Verification items for the finished model (mm, model axes). A direction names the side the tool comes from. Coordinates: 2 decimals unless noted, no trailing zeros. Write each loop counter-clockwise with the first axis right and the second up, starting at its lowest first coordinate (ties: lowest second). Pieces come first, ordered by that corner, then holes. Notation, with made-up numbers: (7.25, -18.75) -> (12.25, -18.75) arc R9 cw to (12.25, -6.75) -> close; hole circle Ø5 at (4, -23.75). An arc over 180 degrees is marked (long way). Write item = value, one per line. Start each with the question number.
(1) Section check A-A (z = 4.25). State how many separate pieces and enclosed holes the cut face has, plus the area to 3 significant figures.
(2) Section check C-C (y = -21). Record the cut outline in (x, z), plus the area to 3 significant figures.
(3) Gauge pin test, flat ends, axial feed: pin 1 Ø1.5 at (y, z) = (-91, 5.5) entering from -X; pin 2 Ø6.5 at (x, y) = (-105.15, -59.25) entering from -Z; pin 3 Ø2 at (x, z) = (-8.5, 5.5) entering from +Y; pin 4 Ø3 at (y, z) = (-80, 5) entering from +X. Record the tip position at first contact, or that the pin passes through.
(4) Section check B-B (x = 103.5). Record the cut outline in (y, z), plus the area to 3 significant figures.
(5) Material ranges on probe 1 along Y at (x, z) = (0.5, 3.75); probe 2 along X at (y, z) = (71, 4); probe 3 along X at (y, z) = (2, 3), recorded low to high. Write a range as [from, to].
(6) Mould release check, pull along Y, two halves, no side actions. Record for faces 3 (the face through (39.956, -35.634, 3.219)), 4 (the face through (21, -19, 0)), 5 (the face through (-103.316, -62.771, 3.219)), 6 (the face through (-94.226, -78.119, 3.131)): released by +Y, released by -Y, zero draft, split by the parting line, or undercut.
(7) Set-up check for faces 1 (the face through (-0.59, 4.46, 3.22)), 2 (the face through (-48.17, -93.9, 3.22)): record each of +Z, -Z, +X, -X, +Y, -Y from which the full face is reachable in a straight line by a thin tool's end or side.
```python
from build123d import *

# Parameters (mm, degrees)
BOSS_EXTRUDE2_DEPTH = 6.35
CUT_EXTRUDE1_DEPTH  = 7.3500001
BOSS_EXTRUDE3_DEPTH = 6.35
SKETCH10_R          = 3.96875
CUT_EXTRUDE2_DEPTH  = 7.35
SKETCH11_R          = 4.5
CUT_EXTRUDE4_DEPTH  = 7.35
BOSS_EXTRUDE4_DEPTH = 6.35
SKETCH13_R          = 1.75
CUT_EXTRUDE5_DEPTH  = 7.35
LPATTERN1_COUNT     = 2
LPATTERN1_PITCH     = 64
SKETCH14_R          = 2.54
CUT_EXTRUDE6_DEPTH  = 7.35
SKETCH15_R          = 1.75
CUT_EXTRUDE7_DEPTH  = 7.35
SKETCH16_R          = 1.75
CUT_EXTRUDE8_DEPTH  = 7.35
SKETCH17_R          = 1.75
CUT_EXTRUDE9_DEPTH  = 7.35
SKETCH19_R          = 3.96875
CUT_EXTRUDE11_DEPTH = 7.35
SKETCH21_R          = 2.54
CUT_EXTRUDE12_DEPTH = 7.35
SKETCH22_R          = 3.96875
CUT_EXTRUDE13_DEPTH = 7.35
SKETCH23_R          = 4.885116726
SKETCH23_R_2        = 5.670398183
BOSS_EXTRUDE5_DEPTH = 6.35
CUT_EXTRUDE14_DEPTH = 7.35
FILLET1_R           = 3.175


with BuildPart() as part:
    # Sketch6 → Boss-Extrude2 (new body)
    with BuildSketch(Plane.XY):
        with BuildLine():
            Line((-68.006850091, -76.67090114), (-109.486767671, -48.656527855))
            Line((-109.486767671, -48.656527855), (-118.371760678, -61.812230963))
            Line((-118.371760678, -61.812230963), (18.447551645, -154.216158235))
            Line((18.447551645, -154.216158235), (135.729459338, 19.43912279))
            Line((135.729459338, 19.43912279), (-1.089852986, 111.843050063))
            Line((-1.089852986, 111.843050063), (-73.946795643, 3.966284577))
            Line((-73.946795643, 3.966284577), (-56.624438948, -7.732749433))
            ThreePointArc((-56.624438948, -7.732749433), (-43.058385537, 37.577891571), (0, 57.15))
            ThreePointArc((0, 57.15), (56.404848571, 31.095576642), (70.829334649, -29.338471048))
            add(Edge.make_bspline(
                [(70.829334649, -29.338471048), (70.811686062, -29.418295928), (70.776015112, -29.578104383), (70.713320217, -29.85478305), (70.619021771, -30.262929245), (70.501052001, -30.762086912), (70.364034474, -31.322191481), (70.199318515, -31.970958926), (70.000453855, -32.723919765), (69.795103485, -33.469783355), (69.582015398, -34.214296028), (69.361377803, -34.956693289), (69.133257682, -35.696762218), (68.838782679, -36.61892651), (68.470566207, -37.720710028), (68.019498024, -38.998776477), (67.474836154, -40.448808619), (66.901337925, -41.887676852), (66.299328392, -43.31485223), (65.669141732, -44.729810424), (65.011119088, -46.132040323), (64.325609411, -47.52103904), (63.612968547, -48.896314904), (62.87355937, -50.257385735), (62.107751613, -51.603779381), (61.315921169, -52.935034173), (60.49845004, -54.250698756), (59.655726138, -55.550331897), (58.571247582, -57.154294757), (57.220953058, -59.045283389), (55.576035723, -61.200397094), (53.604026134, -63.590264702), (51.54329346, -65.904053004), (49.39728314, -68.138962994), (47.169496434, -70.29235602), (44.863486103, -72.361752995), (42.482847363, -74.344831806), (40.031215607, -76.239428526), (36.882516177, -78.494556171), (32.976808929, -81.016011003), (28.250788286, -83.68089187), (21.41551215, -86.919136497), (14.30829026, -89.526654921), (6.996956895, -91.488176442), (-0.451922312, -92.797413176), (-6.61686174, -93.456358442), (-12.81195397, -93.702029749), (-19.009644204, -93.537285056), (-25.183124422, -92.966685286), (-31.306438312, -91.996382122), (-36.598524037, -90.804323442), (-41.072542301, -89.543185606), (-44.752319298, -88.33589156), (-47.664184976, -87.27761875), (-50.541347258, -86.128353728), (-53.381128552, -84.889612663), (-56.180924218, -83.562977818), (-58.593536599, -82.326710176), (-60.633378351, -81.214215821), (-62.313751085, -80.252471782), (-63.646071553, -79.462491566), (-64.966093336, -78.652178853), (-66.222359154, -77.854259082), (-67.143044791, -77.250601571), (-67.736251212, -76.85365602), (-68.006850091, -76.67090114)],
                knots=[0.071020771, 0.071020771, 0.071020771, 0.071020771, 0.071020771, 0.072848477, 0.074676184, 0.07650389, 0.078331597, 0.08198701, 0.085642423, 0.089297836, 0.092953249, 0.096608662, 0.100264075, 0.103919488, 0.107574901, 0.114885727, 0.122196554, 0.12950738, 0.136818214, 0.144129048, 0.151439882, 0.158750716, 0.166061558, 0.173372401, 0.180683243, 0.187994085, 0.195304924, 0.202615763, 0.209926602, 0.217237441, 0.231859103, 0.246480766, 0.261102426, 0.275724085, 0.290345754, 0.304967424, 0.319589099, 0.334210774, 0.348832457, 0.36345414, 0.392697464, 0.421940789, 0.451184112, 0.506140643, 0.535383973, 0.564627303, 0.593870641, 0.623113979, 0.652357319, 0.68160066, 0.710843985, 0.740087309, 0.754708984, 0.769330659, 0.783952333, 0.798574008, 0.813195669, 0.82781733, 0.842438991, 0.849749821, 0.857060652, 0.86437149, 0.871682327, 0.878993165, 0.885158103, 0.885158103, 0.885158103, 0.885158103, 0.885158103], degree=4))
        make_face()
    extrude(amount=BOSS_EXTRUDE2_DEPTH)

    # Sketch8 → Cut-Extrude1 (cut, through all)
    with BuildSketch(Plane.XY.offset(6.35)):
        Polygon((-71.011229489, -93.798205788), (-53.378672597, -90.381637707), (-42.854110111, -97.489632113), (-39.43754203, -115.122189004), align=None)
    extrude(amount=-CUT_EXTRUDE1_DEPTH, mode=Mode.SUBTRACT)

    # Sketch9 → Boss-Extrude3 (add, through all)
    with BuildSketch(Plane.XY.offset(6.35)):
        Polygon((-1.089852986, 111.843050063), (-109.486767671, -48.656527855), (27.332544652, -141.060455127), (135.729459338, 19.43912279), align=None)
    extrude(amount=-BOSS_EXTRUDE3_DEPTH)

    # Sketch10 → Cut-Extrude2 (cut, through all)
    with BuildSketch(Plane.XY.offset(6.35)):
        with Locations((4.996496209, -84.796642912)):
            Circle(SKETCH10_R)
        with Locations((40.816310536, -31.759477627)):
            Circle(SKETCH10_R)
        with Locations((76.636124864, 21.277687659)):
            Circle(SKETCH10_R)
        with Locations((-45.295165913, -45.214466102)):
            Circle(SKETCH10_R)
    extrude(amount=-CUT_EXTRUDE2_DEPTH, mode=Mode.SUBTRACT)

    # Sketch11 → Cut-Extrude4 (cut, through all)
    with BuildSketch(Plane.XY.offset(6.35)):
        Circle(SKETCH11_R)
    extrude(amount=-CUT_EXTRUDE4_DEPTH, mode=Mode.SUBTRACT)

    # Sketch12 → Boss-Extrude4 (add, through all)
    with BuildSketch(Plane.XY.offset(6.35)):
        Polygon((135.729459338, 19.43912279), (67.319803176, 65.641086427), (88.643786393, 97.214773886), (157.053442554, 51.01281025), align=None)
    extrude(amount=-BOSS_EXTRUDE4_DEPTH)

    # Sketch13 → Cut-Extrude5 (cut, through all)
    with BuildSketch(Plane.XY.offset(6.35)):
        with Locations((94.899221836, -29.671127724)):
            Circle(SKETCH13_R)
    cut_extrude5 = extrude(amount=-CUT_EXTRUDE5_DEPTH, mode=Mode.SUBTRACT)

    # LPattern1: Cut-Extrude5 ×2
    with Locations(*[Vector(-0.559684599, -0.828705708, 0) * (i * LPATTERN1_PITCH) for i in range(1, LPATTERN1_COUNT)]):
        add(cut_extrude5, mode=Mode.SUBTRACT)

    # Sketch14 → Cut-Extrude6 (cut, through all)
    with BuildSketch(Plane.XY.offset(6.35)):
        with Locations((71.72703343, -52.635713164)):
            Circle(SKETCH14_R)
        with Locations((35.907219102, -105.67287845)):
            Circle(SKETCH14_R)
        with Locations((115.740620068, 63.589229581)):
            Circle(SKETCH14_R)
    extrude(amount=-CUT_EXTRUDE6_DEPTH, mode=Mode.SUBTRACT)

    # Sketch15 → Cut-Extrude7 (cut, through all)
    with BuildSketch(Plane.XY.offset(6.35)):
        with Locations((-105.147343009, -59.249804902)):
            Circle(SKETCH15_R)
        with Locations((15.885125585, -140.991740566)):
            Circle(SKETCH15_R)
        with Locations((1.472573075, 98.618632394)):
            Circle(SKETCH15_R)
    extrude(amount=-CUT_EXTRUDE7_DEPTH, mode=Mode.SUBTRACT)

    # Sketch16 → Cut-Extrude8 (cut, through all)
    with BuildSketch(Plane.XY.offset(6.35)):
        with Locations((92.060354474, 79.582216994)):
            Circle(SKETCH16_R)
        with Locations((139.420885662, 47.596242169)):
            Circle(SKETCH16_R)
    extrude(amount=-CUT_EXTRUDE8_DEPTH, mode=Mode.SUBTRACT)

    # Sketch17 → Cut-Extrude9 (cut, through all)
    with BuildSketch(Plane.XY.offset(6.35)):
        with Locations((-26.311406216, 17.769986014)):
            Circle(SKETCH17_R)
        with Locations((17.769986014, 26.311406216)):
            Circle(SKETCH17_R)
    extrude(amount=-CUT_EXTRUDE9_DEPTH, mode=Mode.SUBTRACT)

    # Sketch19 → Cut-Extrude11 (cut, through all)
    with BuildSketch(Plane.XY.offset(6.35)):
        with Locations((-65.680233685, -85.904783923)):
            Circle(SKETCH19_R)
    extrude(amount=-CUT_EXTRUDE11_DEPTH, mode=Mode.SUBTRACT)

    # Sketch21 → Cut-Extrude12 (cut, through all)
    with BuildSketch(Plane.XY.offset(6.35)):
        with Locations((-13.666272317, 70.530227577)):
            Circle(SKETCH21_R)
        with Locations((26.00698069, 78.217505758)):
            Circle(SKETCH21_R)
        with Locations((-86.729358658, -71.688795112)):
            Circle(SKETCH21_R)
        with Locations((-8.64928203, -120.590613931)):
            Circle(SKETCH21_R)
    extrude(amount=-CUT_EXTRUDE12_DEPTH, mode=Mode.SUBTRACT)

    # Sketch22 → Cut-Extrude13 (cut, through all)
    with BuildSketch(Plane.XY.offset(6.35)):
        with Locations((-105.147343009, -59.249804902)):
            Circle(SKETCH22_R)
    extrude(amount=-CUT_EXTRUDE13_DEPTH, mode=Mode.SUBTRACT)

    # Sketch23 → Boss-Extrude5 (add, through all)
    with BuildSketch(Plane.XY.offset(6.35)):
        with Locations((-86.729358658, -71.688795112)):
            Circle(SKETCH23_R)
        with Locations((-65.680233685, -85.904783923)):
            Circle(SKETCH23_R_2)
    extrude(amount=-BOSS_EXTRUDE5_DEPTH)

    # Sketch24 → Cut-Extrude14 (cut, through all)
    with BuildSketch(Plane.XY.offset(6.35)):
        Polygon((85.800588631, 93.004948891), (87.167215863, 85.951926135), (71.529628171, 62.797888664), (67.319803176, 65.641086427), align=None)
    extrude(amount=-CUT_EXTRUDE14_DEPTH, mode=Mode.SUBTRACT)

    # Fillet1
    fillet1_edges = [part.edges().sort_by_distance(p)[0] for p in [
        (-1.089852986, 111.843050063, 3.175),
        (18.447551645, -154.216158235, 3.175),
        (-118.371760678, -61.812230963, 3.175),
        (85.800588631, 93.004948891, 3.175),
        (87.167215863, 85.951926135, 3.175),
        (71.529628171, 62.797888664, 3.175),
        (-39.43754203, -115.122189004, 3.175),
        (-71.011229489, -93.798205788, 3.175),
        (-53.378672597, -90.381637707, 3.175),
        (-42.854110111, -97.489632113, 3.175),
        (157.053442554, 51.01281025, 3.175),
        (88.643786393, 97.214773886, 3.175),
    ]]
    fillet(fillet1_edges, radius=FILLET1_R)


solid = part.part
```
Response:
q1.separate_pieces = 1
q1.enclosed_holes = 20
q1.area = 36,700 mm2
q2.outline = (-90.81, 0) -> (108.42, 0) -> (108.42, 6.35) -> (-90.81, 6.35) -> close
q2.area = 1,270 mm2
q3.pin_1 = -76.26
q3.pin_2 = through
q3.pin_3 = 102.35
q3.pin_4 = 69.58
q4.outline = (-28.28, 0) -> (87.18, 0) -> (87.18, 6.35) -> (-28.28, 6.35) -> close
q4.area = 733 mm2
q5.probe_1 = [-142.09, -4.47], [4.47, 97.16], [100.07, 110.52]
q5.probe_2 = [-28.67, -16.16], [-11.17, 59.39], [77.07, 127.46]
q5.probe_3 = [-75.27, -4.03], [4.03, 123.95]
q6.face_3 = undercut
q6.face_4 = zero draft
q6.face_5 = undercut
q6.face_6 = released by -Y
q7.face_1 = +Z, -Z
q7.face_2 = +Z, -Z, -Y
